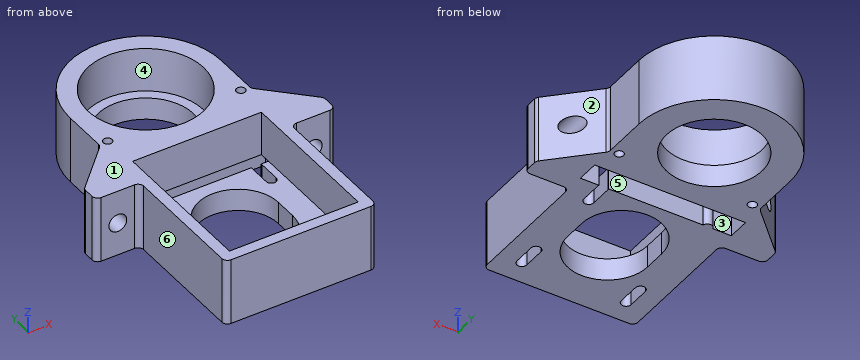
```python
from build123d import *

# Parameters (mm, degrees)
ESQUISSE1_R             = 2
ESQUISSE1_W             = 58
ESQUISSE1_H             = 68
ESQUISSE1_R_2           = 26
BOSS_EXTRU_1_DEPTH      = 20
ESQUISSE1_4_R           = 2
ESQUISSE1_4_R_2         = 21.5
BOSS_EXTRU_2_DEPTH      = 10
ESQUISSE2_R             = 4
ENL_V_MAT_EXTRU_2_DEPTH = 84
CONG_1_R                = 2.5


with BuildPart() as part:
    # Esquisse1 → Boss.-Extru.1 (new body)
    with BuildSketch(Plane.XY):
        with BuildLine():
            Line((34, -109), (34, -49))
            Line((34, -49), (54, -49))
            Line((54, -49), (54, -41))
            Line((54, -41), (34, -21))
            Line((34, -21), (34, 0))
            ThreePointArc((34, 0), (0, 34), (-34, 0))
            Line((-34, 0), (-34, -21))
            Line((-34, -21), (-54, -41))
            Line((-54, -41), (-54, -49))
            Line((-54, -49), (-34, -49))
            Line((-34, -49), (-34, -109))
            Line((-34, -109), (34, -109))
        make_face()
        with Locations((-30, -20)):
            Circle(ESQUISSE1_R, mode=Mode.SUBTRACT)
        with Locations((0, -70)):
            Rectangle(ESQUISSE1_W, ESQUISSE1_H, mode=Mode.SUBTRACT)
        Circle(ESQUISSE1_R_2, mode=Mode.SUBTRACT)
        with Locations((30, -20)):
            Circle(ESQUISSE1_R, mode=Mode.SUBTRACT)
    extrude(amount=BOSS_EXTRU_1_DEPTH)

    # Esquisse1<4> → Boss.-Extru.2 (add)
    with BuildSketch(Plane.XY):
        with BuildLine():
            Line((34, -109), (34, -49))
            Line((34, -49), (54, -49))
            Line((54, -49), (54, -41))
            Line((54, -41), (34, -21))
            Line((34, -21), (34, 0))
            ThreePointArc((34, 0), (0, 34), (-34, 0))
            Line((-34, 0), (-34, -21))
            Line((-34, -21), (-54, -41))
            Line((-54, -41), (-54, -49))
            Line((-54, -49), (-34, -49))
            Line((-34, -49), (-34, -109))
            Line((-34, -109), (34, -109))
        make_face()
        with Locations((-30, -20)):
            Circle(ESQUISSE1_4_R, mode=Mode.SUBTRACT)
        with BuildLine():
            Line((34, -31), (34, -41))
            Line((34, -41), (25.693741097, -41))
            ThreePointArc((25.693741097, -41), (25.735891038, -41.248422445), (25.75, -41.5))
            Line((25.75, -41.5), (25.75, -51.5))
            ThreePointArc((25.75, -51.5), (23.5, -53.75), (21.25, -51.5))
            Line((21.25, -51.5), (21.25, -41.5))
            ThreePointArc((21.25, -41.5), (21.264108962, -41.248422445), (21.306258903, -41))
            Line((21.306258903, -41), (-21.306258903, -41))
            ThreePointArc((-21.306258903, -41), (-23.5, -39.25), (-25.693741097, -41))
            Line((-25.693741097, -41), (-34, -41))
            Line((-34, -41), (-34, -31))
            Line((-34, -31), (34, -31))
        make_face(mode=Mode.SUBTRACT)
        with BuildLine():
            ThreePointArc((18, -75), (0, -93), (-18, -75))
            Line((-18, -75), (-18, -65))
            ThreePointArc((-18, -65), (0, -47), (18, -65))
            Line((18, -65), (18, -75))
        make_face(mode=Mode.SUBTRACT)
        with BuildLine():
            Line((25.75, -88.5), (25.75, -98.5))
            ThreePointArc((25.75, -98.5), (23.5, -100.75), (21.25, -98.5))
            Line((21.25, -98.5), (21.25, -88.5))
            ThreePointArc((21.25, -88.5), (23.5, -86.25), (25.75, -88.5))
        make_face(mode=Mode.SUBTRACT)
        with BuildLine():
            ThreePointArc((-21.25, -98.5), (-23.5, -100.75), (-25.75, -98.5))
            Line((-25.75, -98.5), (-25.75, -88.5))
            ThreePointArc((-25.75, -88.5), (-23.5, -86.25), (-21.25, -88.5))
            Line((-21.25, -88.5), (-21.25, -98.5))
        make_face(mode=Mode.SUBTRACT)
        Circle(ESQUISSE1_4_R_2, mode=Mode.SUBTRACT)
        with Locations((30, -20)):
            Circle(ESQUISSE1_4_R, mode=Mode.SUBTRACT)
    extrude(amount=-BOSS_EXTRU_2_DEPTH)

    # Esquisse2 → Enlèv. mat.-Extru.2 (cut, through all)
    with BuildSketch(Plane.XZ.offset(49)):
        with Locations((44, 5)):
            Circle(ESQUISSE2_R)
        with Locations((-44, 5)):
            Circle(ESQUISSE2_R)
    extrude(amount=-ENL_V_MAT_EXTRU_2_DEPTH, mode=Mode.SUBTRACT)

    # Congé1
    cong_1_edges = [part.edges().sort_by_distance(p)[0] for p in [
        (34, -21, 5),
        (54, -41, 5),
        (54, -49, 5),
        (34, -49, 5),
        (34, -109, 5),
        (-34, -109, 5),
        (-34, -49, 5),
        (-54, -49, 5),
        (-54, -41, 5),
        (-34, -21, 5),
    ]]
    fillet(cong_1_edges, radius=CONG_1_R)


solid = part.part
```
Source: CAD feature listing. Evaluate the final solid. Frame: model axes, mm. Face numbers are marked on the shaded views. A direction names the side the tool comes from. Round coordinates to 2 decimals unless told otherwise and drop trailing zeros. Loops run counter-clockwise (first coordinate to the right, second up) from the corner with the lowest first, then second, coordinate; pieces in that order, holes last.
(1) Pull-direction query (X, two-part tool) for the marked faces 1, 2 and 3; classes: +X half, -X half, draft (parallel to the pull), parting line (faces both ways), or undercut.
From the geometry:
face 1: draft
face 2: +X half
face 3: undercut
(2) Section query C-C (y = -24). Output: boundary loops of the cut face in (x, z), and give its area (3 significant figures).
From the geometry:
outline: (-37, -10) - (37, -10) - (37, 20) - (10, 20) - (10, 0) - (-10, 0) - (-10, 20) - (-37, 20) - close
area: 1,820 mm2
(3) Section query D-D (y = 13). Output: boundary loops of the cut face in (x, z).
From the geometry:
outline: (-31.42, -10) - (-17.12, -10) - (-17.12, 0) - (-22.52, 0) - (-22.52, 20) - (-31.42, 20) - close; (17.12, -10) - (31.42, -10) - (31.42, 20) - (22.52, 20) - (22.52, 0) - (17.12, 0) - close
(4) Section query A-A (x = 44). Output: boundary loops of the cut face in (y, z).
From the geometry:
outline: (-49, -10) - (-31, -10) - (-31, 1) - (-49, 1) - close; (-49, 9) - (-31, 9) - (-31, 20) - (-49, 20) - close
(5) Contact query for flat-ended pins moving along their axis: pin 1 Ø1 at (y, z) = (-77, -3.5) entering from -X; pin 2 Ø6.5 at (x, z) = (-44, 5) entering from -Y; pin 3 Ø1 at (x, z) = (1, -2.5) entering from +Y; pin 4 Ø2 at (x, z) = (-41.5, -6) entering from +Y. Output: stop coordinate, or through.
From the geometry:
pin 1: stops at x = -34
pin 2: passes through
pin 3: stops at y = 34
pin 4: stops at y = -27.5
(6) Material intervals for probe 1 along Y at (x, z) = (0, 7.5); probe 2 along X at (y, z) = (-91, 4.75); probe 3 along Y at (x, z) = (23, -4.5), sorted ascending.
From the geometry:
probe 1: y = -109 to -104, -36 to -26, 26 to 34
probe 2: x = -34 to -29, 29 to 34
probe 3: y = -109 to -100.69, -86.31 to -53.69, -31 to 25.04
(7) Section query B-B (z = 5). Give the number of separate pieces and of enclosed holes in the cut face, and give its area (3 significant figures).
From the geometry:
separate pieces: 3
enclosed holes: 4
area: 3,560 mm2
(8) Access query for the marked faces 4, 5 and 6. Directions: +Z, -Z, +X, -X, +Y, -Y. A direction counts if a zero-diameter tool reaches every point of the face in a straight line with its end or side. Return the directions, or none.
From the geometry:
face 4: +Z
face 5: +Z, -Z
face 6: +Z, -Z, -X, -Y
